Check sheet for the modelled part. Datum: model origin and axes. Units: mm. Face numbers are marked on the shaded views. A direction names the side the tool comes from. Coordinates: 2 decimals unless noted, no trailing zeros. Loops run counter-clockwise (first coordinate to the right, second up) from the corner with the lowest first, then second, coordinate; pieces in that order, holes last. Notation, with made-up numbers: (68.5, 53) - (79.5, 53) arc R19 cw to (79.5, 71) - close; hole circle Ø6 at (1, 18). An arc over 180 degrees is marked (long way). Use a Markdown table: item, result. Add a question column.
1) Draft check along X on the marked faces 4, 5 and 6. Enter one of: pulls with the +X half, pulls with the -X half, needs draft (parallel to the pull), parting line crosses it, or undercut.
2) Sectioned sample at C-C, the plane x = 2. Enter the section's corners in (y, z).
3) Thickness scan on line 1 (Z direction, x = -6.5, y = 3.3); line 2 (X direction, y = 3, z = -8). Record the ranges inside material, lowest first.
4) Sectioned sample at A-A, the plane x = -7.75. Enter the section's corners in (y, z).
5) Go/stop test with a flat-tipped pin: P1, Ø3, axis at y = 1.5, z = 5, coming from the +X side. Record where the tip stops, or that it passes through.
6) Sectioned sample at B-B, the plane z = -0.5. Enter the section's corners in (x, y), then the cut area to 3 significant figures.
7) Tool access check on the marked faces 1, 2 and 3. Record the directions out of +Z, -Z, +X, -X, +Y, -Y that give a thin tool (end or side, any length) a straight path to the whole face; none if there is none.
8) Sectioned sample at D-D, the plane z = -8.25. Enter the section's corners in (x, y), then the cut area to 3 significant figures.
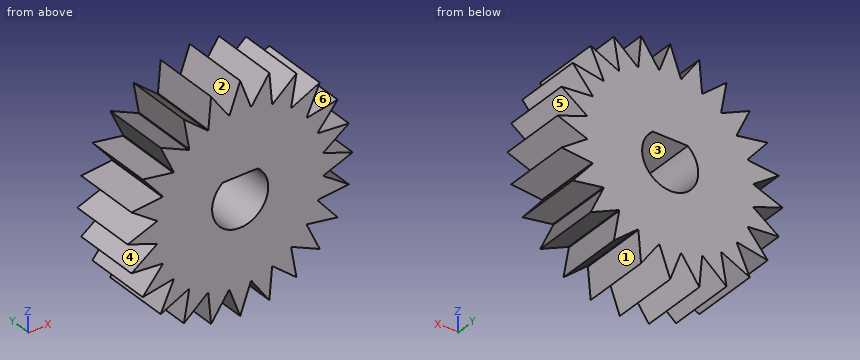
from build123d import *

# Parameters (mm, degrees)
SKETCH_1_R      = 7.5
EXTRUDE_2_DEPTH = 6


with BuildPart() as part:
    # Эскиз1 → Бобышка-Вытянуть2 (new body)
    # profile 1 of 25: a face of its own
    with BuildSketch(Plane(origin=(0, 0, 0), x_dir=(1, 0, 0), z_dir=(0, 1, 0))):
        Circle(SKETCH_1_R)
        with BuildLine():
            Line((-1.564448785, -1.95), (1.564448785, -1.95))
            ThreePointArc((1.564448785, -1.95), (0, 2.5), (-1.564448785, -1.95))
        make_face(mode=Mode.SUBTRACT)
    # profile 2 of 25: a face of its own
    with BuildSketch(Plane(origin=(0, 0, 0), x_dir=(1, 0, 0), z_dir=(0, 1, 0))):
        with BuildLine():
            Line((0, 10.03), (-0.949523561, 7.439650866))
            ThreePointArc((-0.949523561, 7.439650866), (0, 7.5), (0.949523561, 7.439650866))
            Line((0.949523561, 7.439650866), (0, 10.03))
        make_face()
    # profile 3 of 25: a face of its own
    with BuildSketch(Plane(origin=(0, 0, 0), x_dir=(1, 0, 0), z_dir=(0, 1, 0))):
        with BuildLine():
            ThreePointArc((-2.842692663, 6.940396129), (-1.941142838, 7.244443697), (-1.008354003, 7.431905691))
            Line((-1.008354003, 7.431905691), (-2.595955022, 9.688236038))
            Line((-2.595955022, 9.688236038), (-2.842692663, 6.940396129))
        make_face()
    # profile 4 of 25: a face of its own
    with BuildSketch(Plane(origin=(0, 0, 0), x_dir=(1, 0, 0), z_dir=(0, 1, 0))):
        with BuildLine():
            ThreePointArc((-4.542136958, 5.968164865), (-3.75, 6.495190528), (-2.897513908, 6.917688426))
            Line((-2.897513908, 6.917688426), (-5.015, 8.6862348))
            Line((-5.015, 8.6862348), (-4.542136958, 5.968164865))
        make_face()
    # profile 5 of 25: a face of its own
    with BuildSketch(Plane(origin=(0, 0, 0), x_dir=(1, 0, 0), z_dir=(0, 1, 0))):
        with BuildLine():
            ThreePointArc((-5.932042126, 4.589213028), (-5.303300859, 5.303300859), (-4.589213028, 5.932042126))
            Line((-4.589213028, 5.932042126), (-7.092281015, 7.092281015))
            Line((-7.092281015, 7.092281015), (-5.932042126, 4.589213028))
        make_face()
    # profile 6 of 25: a face of its own
    with BuildSketch(Plane(origin=(0, 0, 0), x_dir=(1, 0, 0), z_dir=(0, 1, 0))):
        with BuildLine():
            ThreePointArc((-6.917688426, 2.897513908), (-6.495190528, 3.75), (-5.968164865, 4.542136958))
            Line((-5.968164865, 4.542136958), (-8.6862348, 5.015))
            Line((-8.6862348, 5.015), (-6.917688426, 2.897513908))
        make_face()
    # profile 7 of 25: a face of its own
    with BuildSketch(Plane(origin=(0, 0, 0), x_dir=(1, 0, 0), z_dir=(0, 1, 0))):
        with BuildLine():
            ThreePointArc((-7.431905691, 1.008354003), (-7.244443697, 1.941142838), (-6.940396129, 2.842692663))
            Line((-6.940396129, 2.842692663), (-9.688236038, 2.595955022))
            Line((-9.688236038, 2.595955022), (-7.431905691, 1.008354003))
        make_face()
    # profile 8 of 25: a face of its own
    with BuildSketch(Plane(origin=(0, 0, 0), x_dir=(1, 0, 0), z_dir=(0, 1, 0))):
        with BuildLine():
            ThreePointArc((-7.439650866, -0.949523561), (-7.5, 0), (-7.439650866, 0.949523561))
            Line((-7.439650866, 0.949523561), (-10.03, 0))
            Line((-10.03, 0), (-7.439650866, -0.949523561))
        make_face()
    # profile 9 of 25: a face of its own
    with BuildSketch(Plane(origin=(0, 0, 0), x_dir=(1, 0, 0), z_dir=(0, 1, 0))):
        with BuildLine():
            ThreePointArc((-6.940396129, -2.842692663), (-7.244443697, -1.941142838), (-7.431905691, -1.008354003))
            Line((-7.431905691, -1.008354003), (-9.688236038, -2.595955022))
            Line((-9.688236038, -2.595955022), (-6.940396129, -2.842692663))
        make_face()
    # profile 10 of 25: a face of its own
    with BuildSketch(Plane(origin=(0, 0, 0), x_dir=(1, 0, 0), z_dir=(0, 1, 0))):
        with BuildLine():
            ThreePointArc((-5.968164865, -4.542136958), (-6.495190528, -3.75), (-6.917688426, -2.897513908))
            Line((-6.917688426, -2.897513908), (-8.6862348, -5.015))
            Line((-8.6862348, -5.015), (-5.968164865, -4.542136958))
        make_face()
    # profile 11 of 25: a face of its own
    with BuildSketch(Plane(origin=(0, 0, 0), x_dir=(1, 0, 0), z_dir=(0, 1, 0))):
        with BuildLine():
            ThreePointArc((-4.589213028, -5.932042126), (-5.303300859, -5.303300859), (-5.932042126, -4.589213028))
            Line((-5.932042126, -4.589213028), (-7.092281015, -7.092281015))
            Line((-7.092281015, -7.092281015), (-4.589213028, -5.932042126))
        make_face()
    # profile 12 of 25: a face of its own
    with BuildSketch(Plane(origin=(0, 0, 0), x_dir=(1, 0, 0), z_dir=(0, 1, 0))):
        with BuildLine():
            ThreePointArc((-2.897513908, -6.917688426), (-3.75, -6.495190528), (-4.542136958, -5.968164865))
            Line((-4.542136958, -5.968164865), (-5.015, -8.6862348))
            Line((-5.015, -8.6862348), (-2.897513908, -6.917688426))
        make_face()
    # profile 13 of 25: a face of its own
    with BuildSketch(Plane(origin=(0, 0, 0), x_dir=(1, 0, 0), z_dir=(0, 1, 0))):
        with BuildLine():
            ThreePointArc((-1.008354003, -7.431905691), (-1.941142838, -7.244443697), (-2.842692663, -6.940396129))
            Line((-2.842692663, -6.940396129), (-2.595955022, -9.688236038))
            Line((-2.595955022, -9.688236038), (-1.008354003, -7.431905691))
        make_face()
    # profile 14 of 25: a face of its own
    with BuildSketch(Plane(origin=(0, 0, 0), x_dir=(1, 0, 0), z_dir=(0, 1, 0))):
        with BuildLine():
            ThreePointArc((0.949523561, -7.439650866), (0, -7.5), (-0.949523561, -7.439650866))
            Line((-0.949523561, -7.439650866), (0, -10.03))
            Line((0, -10.03), (0.949523561, -7.439650866))
        make_face()
    # profile 15 of 25: a face of its own
    with BuildSketch(Plane(origin=(0, 0, 0), x_dir=(1, 0, 0), z_dir=(0, 1, 0))):
        with BuildLine():
            Line((2.595955022, -9.688236038), (2.842692663, -6.940396129))
            ThreePointArc((2.842692663, -6.940396129), (1.941142838, -7.244443697), (1.008354003, -7.431905691))
            Line((1.008354003, -7.431905691), (2.595955022, -9.688236038))
        make_face()
    # profile 16 of 25: a face of its own
    with BuildSketch(Plane(origin=(0, 0, 0), x_dir=(1, 0, 0), z_dir=(0, 1, 0))):
        with BuildLine():
            Line((5.015, -8.6862348), (4.542136958, -5.968164865))
            ThreePointArc((4.542136958, -5.968164865), (3.75, -6.495190528), (2.897513908, -6.917688426))
            Line((2.897513908, -6.917688426), (5.015, -8.6862348))
        make_face()
    # profile 17 of 25: a face of its own
    with BuildSketch(Plane(origin=(0, 0, 0), x_dir=(1, 0, 0), z_dir=(0, 1, 0))):
        with BuildLine():
            Line((7.092281015, -7.092281015), (5.932042126, -4.589213028))
            ThreePointArc((5.932042126, -4.589213028), (5.303300859, -5.303300859), (4.589213028, -5.932042126))
            Line((4.589213028, -5.932042126), (7.092281015, -7.092281015))
        make_face()
    # profile 18 of 25: a face of its own
    with BuildSketch(Plane(origin=(0, 0, 0), x_dir=(1, 0, 0), z_dir=(0, 1, 0))):
        with BuildLine():
            Line((8.6862348, -5.015), (6.917688426, -2.897513908))
            ThreePointArc((6.917688426, -2.897513908), (6.495190528, -3.75), (5.968164865, -4.542136958))
            Line((5.968164865, -4.542136958), (8.6862348, -5.015))
        make_face()
    # profile 19 of 25: a face of its own
    with BuildSketch(Plane(origin=(0, 0, 0), x_dir=(1, 0, 0), z_dir=(0, 1, 0))):
        with BuildLine():
            Line((9.688236038, -2.595955022), (7.431905691, -1.008354003))
            ThreePointArc((7.431905691, -1.008354003), (7.244443697, -1.941142838), (6.940396129, -2.842692663))
            Line((6.940396129, -2.842692663), (9.688236038, -2.595955022))
        make_face()
    # profile 20 of 25: a face of its own
    with BuildSketch(Plane(origin=(0, 0, 0), x_dir=(1, 0, 0), z_dir=(0, 1, 0))):
        with BuildLine():
            Line((10.03, 0), (7.439650866, 0.949523561))
            ThreePointArc((7.439650866, 0.949523561), (7.484897511, 0.475719721), (7.5, 0))
            ThreePointArc((7.5, 0), (7.484897511, -0.475719721), (7.439650866, -0.949523561))
            Line((7.439650866, -0.949523561), (10.03, 0))
        make_face()
    # profile 21 of 25: a face of its own
    with BuildSketch(Plane(origin=(0, 0, 0), x_dir=(1, 0, 0), z_dir=(0, 1, 0))):
        with BuildLine():
            Line((9.688236038, 2.595955022), (6.940396129, 2.842692663))
            ThreePointArc((6.940396129, 2.842692663), (7.244443697, 1.941142838), (7.431905691, 1.008354003))
            Line((7.431905691, 1.008354003), (9.688236038, 2.595955022))
        make_face()
    # profile 22 of 25: a face of its own
    with BuildSketch(Plane(origin=(0, 0, 0), x_dir=(1, 0, 0), z_dir=(0, 1, 0))):
        with BuildLine():
            Line((8.6862348, 5.015), (5.968164865, 4.542136958))
            ThreePointArc((5.968164865, 4.542136958), (6.495190528, 3.75), (6.917688426, 2.897513908))
            Line((6.917688426, 2.897513908), (8.6862348, 5.015))
        make_face()
    # profile 23 of 25: a face of its own
    with BuildSketch(Plane(origin=(0, 0, 0), x_dir=(1, 0, 0), z_dir=(0, 1, 0))):
        with BuildLine():
            Line((7.092281015, 7.092281015), (4.589213028, 5.932042126))
            ThreePointArc((4.589213028, 5.932042126), (5.303300859, 5.303300859), (5.932042126, 4.589213028))
            Line((5.932042126, 4.589213028), (7.092281015, 7.092281015))
        make_face()
    # profile 24 of 25: a face of its own
    with BuildSketch(Plane(origin=(0, 0, 0), x_dir=(1, 0, 0), z_dir=(0, 1, 0))):
        with BuildLine():
            Line((5.015, 8.6862348), (2.897513908, 6.917688426))
            ThreePointArc((2.897513908, 6.917688426), (3.75, 6.495190528), (4.542136958, 5.968164865))
            Line((4.542136958, 5.968164865), (5.015, 8.6862348))
        make_face()
    # profile 25 of 25: a face of its own
    with BuildSketch(Plane(origin=(0, 0, 0), x_dir=(1, 0, 0), z_dir=(0, 1, 0))):
        with BuildLine():
            Line((2.595955022, 9.688236038), (1.008354003, 7.431905691))
            ThreePointArc((1.008354003, 7.431905691), (1.941142838, 7.244443697), (2.842692663, 6.940396129))
            Line((2.842692663, 6.940396129), (2.595955022, 9.688236038))
        make_face()
    extrude(amount=EXTRUDE_2_DEPTH)


solid = part.part
Solved:
| question | item | result |
|---|---|---|
| 1 | face 4 | pulls with the -X half |
| 1 | face 5 | pulls with the +X half |
| 1 | face 6 | undercut |
| 2 | outline | (0, -8.84) - (6, -8.84) - (6, -1.5) - (0, -1.5) - close; (0, 1.5) - (6, 1.5) - (6, 8.84) - (0, 8.84) - close |
| 3 | line 1 | z = -6.82 to -5.81, -4.63 to 4.63, 5.81 to 6.82 |
| 3 | line 2 | x = -4.9 to -4.19, -2.75 to -1.41, -0.74 to 0.74, 1.41 to 2.75, 4.19 to 4.9 |
| 4 | outline | (0, -4.85) - (6, -4.85) - (6, -3.89) - (0, -3.89) - close; (0, -2.77) - (6, -2.77) - (6, -1.23) - (0, -1.23) - close; (0, -0.84) - (6, -0.84) - (6, 0.84) - (0, 0.84) - close; (0, 1.23) - (6, 1.23) - (6, 2.77) - (0, 2.77) - close; (0, 3.89) - (6, 3.89) - (6, 4.85) - (0, 4.85) - close |
| 5 | P1 | stops at x = 8.69 |
| 6 | outline | (-8.67, 0) - (-2.45, 0) - (-2.45, 6) - (-8.67, 6) - close; (2.45, 0) - (8.67, 0) - (8.67, 6) - (2.45, 6) - close |
| 6 | area | 74.6 mm2 |
| 7 | face 1 | -Z, +Y, -Y |
| 7 | face 2 | +Z, +Y, -Y |
| 7 | face 3 | +Y, -Y |
| 8 | outline | (-4.94, 0) - (-4.49, 0) - (-4.49, 6) - (-4.94, 6) - close; (-2.73, 0) - (-1.58, 0) - (-1.58, 6) - (-2.73, 6) - close; (-0.65, 0) - (0.65, 0) - (0.65, 6) - (-0.65, 6) - close; (1.58, 0) - (2.73, 0) - (2.73, 6) - (1.58, 6) - close; (4.49, 0) - (4.94, 0) - (4.94, 6) - (4.49, 6) - close |
| 8 | area | 26.9 mm2 |
